Build history of the part. All positions in model axes, mm. Round coordinates to 2 decimals unless told otherwise and drop trailing zeros. Loops run counter-clockwise (first coordinate to the right, second up) from the corner with the lowest first, then second, coordinate; pieces in that order, holes last. Notation, with made-up numbers: M 66,-15.5 L 76,-15.5 A22 ccw 76,5.5 Z; hole C 15,54 d2. An arc over 180 degrees is marked long. One line per item, written item: value.
Autodesk Inventor part; units mm, degrees
ref_plane "Work Plane1" through (0, 0, 20.25) normal (0, 0, 1) x (1, 0, 0)
ref_plane "YZ Plane" through (0, 0, 0) normal (1, 0, 0) x (0, 1, 0)
ref_plane "XZ Plane" through (0, 0, 0) normal (0, 1, 0) x (-1, 0, 0)
sketch "Sketch1" plane through (0, 0, 0) normal (0, 0, 1) x (1, 0, 0)
  circle A0 centre (0, 0) radius 21.2375
  circle A1 centre (0, 0) radius 20.2375
  dimension "d0" = 42.475
  dimension "d1" = 1
extrude "Extrusion1" add sketch "Sketch1" along normal mid plane 27.5
sketch "Sketch2" plane through (0, 0, 13.75) normal (0, 0, 1) x (1, 0, 0)
  circle A0 centre (0, 0) radius 21.2375
  circle A1 centre (0, 0) radius 20.2375
  line L0 (-3.925, 20.8717) -> (-3.925, 19.8532)
  line L1 (3.925, 20.8717) -> (3.925, 19.8532)
  point P0 (0, 13.5869)
  dimension "d4" = 7.85
extrude "Extrusion2" add sketch "Sketch2" along normal blind 6.5 contours L1 A1 L0 A0 picked at (3.0552, 20.3065)
pattern_circular "Circular Pattern1" count 3 over 360 about axis through (0, 0, -10) along (0, 0, 1) of "Extrusion2"
sketch "Sketch3" plane through (0, 0, 0) normal (0, 0, 1) x (1, 0, 0)
  point P0 (0, 0)
ref_plane "Work Plane1" through (0, 0, 20.25) normal (0, 0, 1) x (1, 0, 0)
properties part number "Inner part of servo motor" material "Aluminum 6061-AHC"
Item 1: Slice it at C-C, the plane z = 18.5. Give the cut face in (x, y) (1 decimal), and give its area (3 significant figures).
Check values:
outline: M -20,-7 A21.2 ccw -16.1,-13.8 L -15.2,-13.3 A20.2 cw -19.2,-6.5 Z; M -3.9,19.9 A20.2 cw 3.9,19.9 L 3.9,20.9 A21.2 ccw -3.9,20.9 Z; M 15.2,-13.3 L 16.1,-13.8 A21.2 ccw 20,-7 L 19.2,-6.5 A20.2 cw Z
area: 23.7 mm2
Item 2: Drop flat-ended pins along their axis: P1, Ø1, axis at y = -3.5, z = 9, coming from the -X side; P2, Ø3, axis at y = 7, z = 14.5, coming from the -X side; P3, Ø2, axis at y = -8.5, z = -7.5, coming from the +X side. Give the stop position or say it passes through.
Check values:
P1: stops at x = -21.02
P2: stops at x = -20.46
P3: stops at x = 19.87
Item 3: Wall check: line 1 along X through (y, z) = (0, 8); line 2 along X through (y, z) = (18, -11.5). Give the ranges that are in metal, low to high.
Check values:
line 1: x = -21.24 to -20.24, 20.24 to 21.24
line 2: x = -11.27 to -9.25, 9.25 to 11.27
Item 4: Pull direction Y, two halves, no side cores. Call faces 1 (the face through (-20.218, -0.89, -0.766)), 2 (the face through (19, -8, -13.75)): pulls with the +Y half, pulls with the -Y half, needs draft (parallel to the pull), parting line crosses it, or undercut.
Check values:
face 1: undercut
face 2: needs draft
Item 5: Slice it at B-B, the plane y = 0. Give the cut face in (x, z), and give its area (3 significant figures).
Check values:
outline: M -21.24,-13.75 L -20.24,-13.75 L -20.24,13.75 L -21.24,13.75 Z; M 20.24,-13.75 L 21.24,-13.75 L 21.24,13.75 L 20.24,13.75 Z
area: 55.0 mm2
Item 6: Slice it at D-D, the plane z = -8.5. Give the cut face in (x, y) (1 decimal), and give its area (3 significant figures).
Check values:
outline: C 0,0 d42.5; hole C 0,0 d40.5
area: 130 mm2
Item 7: Slice it at A-A, the plane x = 0. Give the cut face in (y, z), and give its area (3 significant figures).
Check values:
outline: M -21.24,-13.75 L -20.24,-13.75 L -20.24,13.75 L -21.24,13.75 Z; M 20.24,-13.75 L 21.24,-13.75 L 21.24,20.25 L 20.24,20.25 Z
area: 61.5 mm2
